Input: dimensioned drawing with shaded views. Units: mm. Origin: part minimum x, y, z. A direction names the side the tool comes from. Give positions to 0.01 mm unless a question says otherwise; leave off trailing zeros. Write each loop counter-clockwise with the first axis right and the second up, starting at its lowest first coordinate (ties: lowest second). Pieces come first, ordered by that corner, then holes. Notation, with made-up numbers: (-5.5, 79.5) -> (49.5, 79.5) arc R31 ccw to (49.5, 108.5) -> close; hole circle Ø2 at (13, 9.5). An arc over 180 degrees is marked (long way). Answer as a JSON object with one key per item and string values.
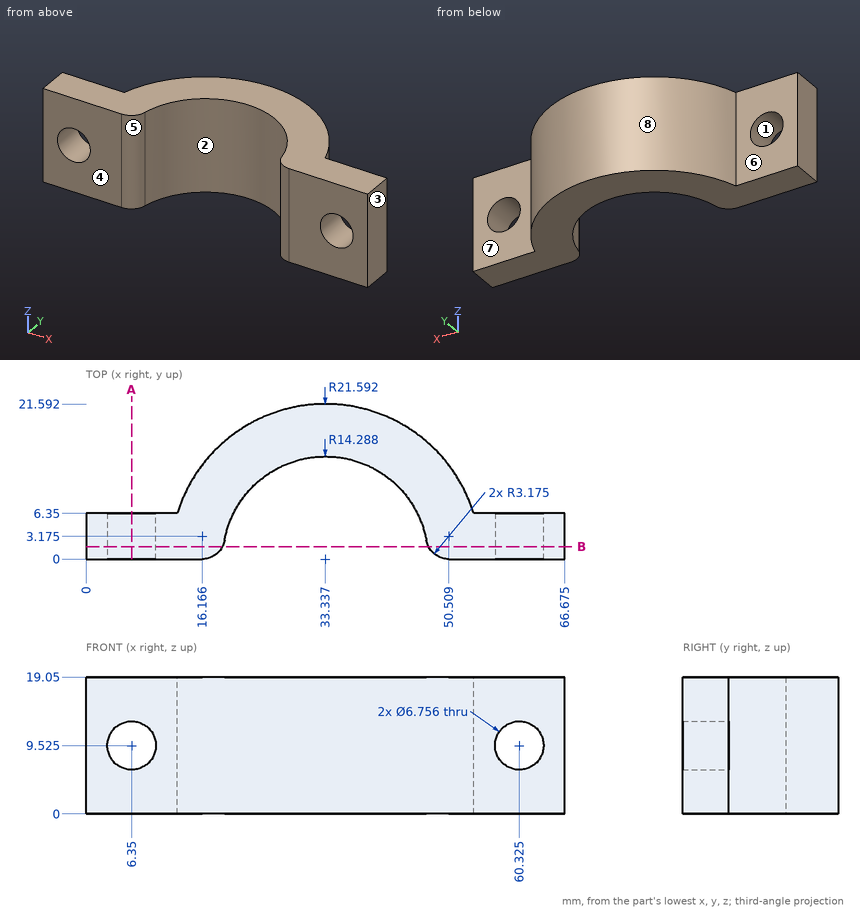
Q1. First-contact query: P1, Ø4, axis at x = 6.35, z = 9.525, coming from the -Y side; P2, Ø3, axis at y = 15, z = 16.5, coming from the +X side; P3, Ø6.5, axis at x = 4.5, z = 12.5, coming from the +Y side; P4, Ø1.5, axis at x = 22.5, z = 9.5, coming from the +Y side. Flat tips, straight axial feed; report the tip coordinate or a pass-through.
Values:
{"P1": "through", "P2": "x = 50.19", "P3": "y = 6.35", "P4": "y = 19.09"}
Q2. Cut plane A-A (x = 6.35). Return the cut outline in (y, z).
Values:
{"outline": "(0, 0) -> (6.35, 0) -> (6.35, 6.15) -> (0, 6.15) -> close; (0, 12.9) -> (6.35, 12.9) -> (6.35, 19.05) -> (0, 19.05) -> close"}
Q3. Cut plane B-B (y = 1.75). State how many separate pieces and enclosed holes the cut face has.
Values:
{"separate pieces": "2", "enclosed holes": "2"}
Q4. Material intervals for L1, parallel to X at y = 3.5, z = 11.25 (1 decimal); L2, parallel to X at y = 1, z = 7.5 (1 decimal); L3, parallel to Y at x = 5, z = 15, sorted ascending. Write a range as from..to.
Values:
{"L1": "0..3.4, 9.3..19.5, 47.2..57.4, 63.2..66.7", "L2": "0..3.6, 9.1..18.5, 48.2..57.6, 63..66.7", "L3": "0..6.35"}
Q5. Mould query, pull axis X, two halves, no side actions, for the marked faces 1, 2, 3 and 4. Classes: pulls with the +X half, pulls with the -X half, needs draft (parallel to the pull), parting line crosses it, or undercut.
Values:
{"face 1": "undercut", "face 2": "undercut", "face 3": "pulls with the +X half", "face 4": "needs draft"}
Q6. Set-up query: the marked faces 5, 6, 7 and 8. Return all of +Z, -Z, +X, -X, +Y, -Y with unobstructed straight access to the full face (end or side cutting, diameter ignored); none if empty.
Values:
{"face 5": "+Z, -Z, -Y", "face 6": "+Z, -Z, -X, +Y", "face 7": "+Z, -Z, +X, +Y", "face 8": "+Z, -Z, +Y"}
